```python
from build123d import *

# Parameters (mm, degrees)
F0_R     = 3
F1_DEPTH = 1
F3_DEPTH = 1
F5_DEPTH = 1
F6_R     = 1.5
F7_DEPTH = 1


with BuildPart() as f1:
    # F0 (on Top) → F1 (new body)
    with BuildSketch(Plane.XY):
        Polygon((68.5, -40), (78.5, -40), (78.5, 40), (33.5, 40), (25.5, 16), (-58.5, 16), (-66.5, 40), (-78.5, 40), (-78.5, -40), (8.5, -40), (8.5, 0), (68.5, 0), align=None)
        with Locations((-8.5, -17)):
            Circle(F0_R, mode=Mode.SUBTRACT)
    extrude(amount=F1_DEPTH)

    # F2 (on face) → F3 (join)
    with BuildSketch(Plane(origin=(-78.5, 0, 0), x_dir=(0, -1, 0), z_dir=(-1, 0, 0))):
        with BuildLine():
            Line((-40, 1), (40, 1))
            Line((40, 1), (40, 10))
            Line((40, 10), (19.787322, 15.05317))
            ThreePointArc((19.787322, 15.05317), (17.058973, 16.826821), (16, 19.903882))
            Line((16, 19.903882), (16, 58.928932))
            ThreePointArc((16, 58.928932), (16.380602, 60.842349), (17.464466, 62.464466))
            Line((17.464466, 62.464466), (40, 85))
            Line((40, 85), (40, 110))
            Line((40, 110), (-30, 110))
            Line((-30, 110), (-30, 10))
            Line((-30, 10), (-40, 10))
            Line((-40, 10), (-40, 1))
        make_face()
        with BuildLine():
            ThreePointArc((-22, 55), (-20.535534, 58.535534), (-17, 60))
            Line((-17, 60), (3, 60))
            ThreePointArc((3, 60), (6.535534, 58.535534), (8, 55))
            Line((8, 55), (8, 15))
            ThreePointArc((8, 15), (6.535534, 11.464466), (3, 10))
            Line((3, 10), (-17, 10))
            ThreePointArc((-17, 10), (-20.535534, 11.464466), (-22, 15))
            Line((-22, 15), (-22, 55))
        make_face(mode=Mode.SUBTRACT)
        with BuildLine():
            ThreePointArc((17.32233, 95.606602), (21.941728, 92.520019), (20.857864, 87.071068))
            Line((20.857864, 87.071068), (6.857864, 73.071068))
            ThreePointArc((6.857864, 73.071068), (5.235748, 71.987204), (3.32233, 71.606602))
            Line((3.32233, 71.606602), (-10.606602, 71.606602))
            ThreePointArc((-10.606602, 71.606602), (-14.142136, 73.071068), (-15.606602, 76.606602))
            Line((-15.606602, 76.606602), (-15.606602, 90.606602))
            ThreePointArc((-15.606602, 90.606602), (-14.142136, 94.142136), (-10.606602, 95.606602))
            Line((-10.606602, 95.606602), (17.32233, 95.606602))
        make_face(mode=Mode.SUBTRACT)
    extrude(amount=-F3_DEPTH)

    # F4 (on face) → F5 (join)
    with BuildSketch(Plane.YZ.offset(78.5)):
        with BuildLine():
            Line((-40, 0), (40, 0))
            Line((40, 0), (40, 10))
            Line((40, 10), (30, 10))
            Line((30, 10), (30, 110))
            Line((30, 110), (-40, 110))
            Line((-40, 110), (-40, 85))
            Line((-40, 85), (-17.464466, 62.464466))
            ThreePointArc((-17.464466, 62.464466), (-16.380602, 60.842349), (-16, 58.928932))
            Line((-16, 58.928932), (-16, 19.903882))
            ThreePointArc((-16, 19.903882), (-17.058973, 16.826821), (-19.787322, 15.05317))
            Line((-19.787322, 15.05317), (-40, 10))
            Line((-40, 10), (-40, 0))
        make_face()
        with BuildLine():
            Line((-3, 60), (17, 60))
            ThreePointArc((17, 60), (20.535534, 58.535534), (22, 55))
            Line((22, 55), (22, 15))
            ThreePointArc((22, 15), (20.535534, 11.464466), (17, 10))
            Line((17, 10), (-3, 10))
            ThreePointArc((-3, 10), (-6.535534, 11.464466), (-8, 15))
            Line((-8, 15), (-8, 55))
            ThreePointArc((-8, 55), (-6.535534, 58.535534), (-3, 60))
        make_face(mode=Mode.SUBTRACT)
        with BuildLine():
            Line((-6.857864, 73.071068), (-20.857864, 87.071068))
            ThreePointArc((-20.857864, 87.071068), (-21.941728, 92.520019), (-17.32233, 95.606602))
            Line((-17.32233, 95.606602), (10.606602, 95.606602))
            ThreePointArc((10.606602, 95.606602), (14.142136, 94.142136), (15.606602, 90.606602))
            Line((15.606602, 90.606602), (15.606602, 76.606602))
            ThreePointArc((15.606602, 76.606602), (14.142136, 73.071068), (10.606602, 71.606602))
            Line((10.606602, 71.606602), (-3.32233, 71.606602))
            ThreePointArc((-3.32233, 71.606602), (-5.235748, 71.987204), (-6.857864, 73.071068))
        make_face(mode=Mode.SUBTRACT)
    extrude(amount=-F5_DEPTH)

    # F6 (on face) → F7 (join)
    with BuildSketch(Plane.XY.offset(110)):
        with BuildLine():
            Line((77.5, 30), (77.5, -40))
            Line((77.5, -40), (92.5, -40))
            ThreePointArc((92.5, -40), (96.035534, -38.535534), (97.5, -35))
            Line((97.5, -35), (97.5, 25))
            ThreePointArc((97.5, 25), (96.035534, 28.535534), (92.5, 30))
            Line((92.5, 30), (77.5, 30))
        make_face()
        with Locations((91, -25.5)):
            Circle(F6_R, mode=Mode.SUBTRACT)
        with Locations((91, 10.5)):
            Circle(F6_R, mode=Mode.SUBTRACT)
        with BuildLine():
            ThreePointArc((-92.5, 30), (-96.035534, 28.535534), (-97.5, 25))
            Line((-97.5, 25), (-97.5, -35))
            ThreePointArc((-97.5, -35), (-96.035534, -38.535534), (-92.5, -40))
            Line((-92.5, -40), (-77.5, -40))
            Line((-77.5, -40), (-77.5, 30))
            Line((-77.5, 30), (-92.5, 30))
        make_face()
        with Locations((-91, -25.5)):
            Circle(F6_R, mode=Mode.SUBTRACT)
        with Locations((-91, 10.5)):
            Circle(F6_R, mode=Mode.SUBTRACT)
    extrude(amount=F7_DEPTH)


solid = f1.part
```
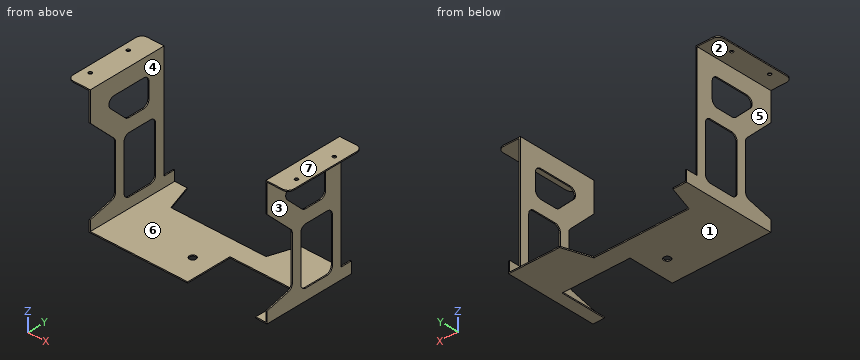
Design review of the part built by this model. Coordinates are the model's own, in mm. Face numbers are marked on the shaded views. A direction names the side the tool comes from. Give positions to 0.01 mm unless a question says otherwise; leave off trailing zeros. Loops run counter-clockwise (first coordinate to the right, second up) from the corner with the lowest first, then second, coordinate; pieces in that order, holes last. Notation, with made-up numbers: (32.5, 77.5) -> (86.5, 77.5) arc R24 ccw to (86.5, 91.5) -> close; hole circle Ø1 at (19.5, 15.5). An arc over 180 degrees is marked (long way). Write each question's results on one line, items separated by ' | '.
Q1. Wall thickness on L1, parallel to Y at x = 91, z = 110.75; L2, parallel to X at y = -34, z = 87.5; L3, parallel to Y at x = -8.5, z = 0.25: over which ranges is each line inside the solid? List them lowest first.
Reply:
L1: y = -40 to -27, -24 to 9, 12 to 30 | L2: x = -78.5 to -77.5, 77.5 to 78.5 | L3: y = -40 to -20, -14 to 16
Q2. Take a section at A-A, the plane y = -30. Write out the cut boundary in (x, z), plus the area to 3 significant figures.
Reply:
outline: (-97.5, 110) -> (-78.5, 110) -> (-78.5, 75) -> (-77.5, 75) -> (-77.5, 111) -> (-97.5, 111) -> close; (-78.5, 0) -> (8.5, 0) -> (8.5, 1) -> (-77.5, 1) -> (-77.5, 12.5) -> (-78.5, 12.5) -> close; (68.5, 0) -> (78.5, 0) -> (78.5, 12.5) -> (77.5, 12.5) -> (77.5, 1) -> (68.5, 1) -> close; (77.5, 75) -> (78.5, 75) -> (78.5, 110) -> (97.5, 110) -> (97.5, 111) -> (77.5, 111) -> close | area: 230 mm²
Q3. Machinability: for the marked faces 1, 2, 3 and 4, which of the approach directions +Z, -Z, +X, -X, +Y, -Y give a long, thin tool a straight path to every point of the face, cutting with its end or side? Answer none if there is none.
Reply:
face 1: -Z, +X, -X, +Y, -Y | face 2: -Z, -X, +Y, -Y | face 3: -Z, +X, +Y, -Y | face 4: +Z, +Y, -Y
Q4. Take a section at B-B, the plane y = 34.5. Write out the cut boundary in (x, z).
Reply:
outline: (-78.5, 0) -> (-64.67, 0) -> (-64.67, 1) -> (-77.5, 1) -> (-77.5, 10) -> (-78.5, 10) -> close; (31.67, 0) -> (78.5, 0) -> (78.5, 10) -> (77.5, 10) -> (77.5, 1) -> (31.67, 1) -> close
Q5. Take a section at D-D, the plane x = 43. Write out the cut boundary in (y, z).
Reply:
outline: (0, 0) -> (40, 0) -> (40, 1) -> (0, 1) -> close
Q6. Take a section at C-C, the plane x = -41. Write out the cut boundary in (y, z), plus the area to 3 significant figures.
Reply:
outline: (-40, 0) -> (16, 0) -> (16, 1) -> (-40, 1) -> close | area: 56.0 mm²
Q7. The part is to be moulded in two halves that separate along X. For the marked faces 5, 6 and 7, say which applies: +X half, -X half, draft (parallel to the pull), parting line (faces both ways), or undercut.
Reply:
face 5: -X half | face 6: undercut | face 7: draft
Q8. For pin 1 Ø0.8 at (x, z) = (-78, 26.5) entering from +Y; pin 2 Ø5 at (y, z) = (13.5, 59) entering from -X; pin 3 Ø0.8 at (x, z) = (-78, 84.5) entering from -Y, all flat-tipped, find the tip position at first contact; note any pin that passes through.
Reply:
pin 1: stops at y = 30 | pin 2: stops at x = -78.5 | pin 3: stops at y = -39.9
